Design review of the part built by this model. Coordinates are the model's own, in mm. A direction names the side the tool comes from. Coordinates: 2 decimals unless noted, no trailing zeros. Order: outer loops, then holes, each group sorted by start corner. A loop starts at its lowest first (then second) coordinate and runs counter-clockwise, first axis right, second up. Notation, with made-up numbers: M 53,51 L 107,51 A22 ccw 107,58 Z; hole C 35.5,-28.5 d7. An arc over 180 degrees is marked long. Answer as a JSON object with one key per item and string values.
from build123d import *

# Parameters (mm, degrees)
BOSS_EXTRUDE1_DEPTH     = 150
CUT_EXTRUDE1_DEPTH      = 173.409396496
CUT_EXTRUDE1_DEPTH_BACK = 173.409396496
SKETCH3_OUTSIDE_W       = 197.344
SKETCH3_OUTSIDE_H       = 197.344
BOSS_EXTRUDE2_START     = -80
BOSS_EXTRUDE2_DEPTH     = 80


with BuildPart() as part:
    # Sketch1 → Boss-Extrude1 (new body)
    with BuildSketch(Plane(origin=(0, 0, 0), x_dir=(1, 0, 0), z_dir=(0, 1, 0))):
        with BuildLine():
            Line((-45, -40), (45, -40))
            ThreePointArc((45, -40), (66.213203436, -31.213203436), (75, -10))
            Line((75, -10), (75, 10))
            ThreePointArc((75, 10), (66.213203436, 31.213203436), (45, 40))
            Line((45, 40), (-45, 40))
            ThreePointArc((-45, 40), (-66.213203436, 31.213203436), (-75, 10))
            Line((-75, 10), (-75, -10))
            ThreePointArc((-75, -10), (-66.213203436, -31.213203436), (-45, -40))
        make_face()
    extrude(amount=BOSS_EXTRUDE1_DEPTH)

    # Sketch3 outside → Cut-Extrude1 (cut, two sides: drawn at the far end of the back side and taken through both)
    with BuildSketch(Plane.XY.offset(-CUT_EXTRUDE1_DEPTH_BACK)):
        with Locations((0, 75)):
            Rectangle(SKETCH3_OUTSIDE_W, SKETCH3_OUTSIDE_H)
        with BuildLine():
            Line((-75, 150), (-75, 0))
            Line((-75, 0), (75, 0))
            Line((75, 0), (75, 150))
            ThreePointArc((75, 150), (0, 116.143782777), (-75, 150))
        make_face(mode=Mode.SUBTRACT)
    extrude(amount=CUT_EXTRUDE1_DEPTH + CUT_EXTRUDE1_DEPTH_BACK, mode=Mode.SUBTRACT)

    # Sketch6 → Boss-Extrude2 (add)
    with BuildSketch(Plane.XY.offset(40).offset(BOSS_EXTRUDE2_START)):
        with BuildLine():
            Line((-45, 126.840927279), (-45, 156.143782777))
            ThreePointArc((-45, 156.143782777), (0, 141.143782777), (45, 156.143782777))
            Line((45, 156.143782777), (45, 126.840927279))
            ThreePointArc((45, 126.840927279), (0, 116.143782777), (-45, 126.840927279))
        make_face()
    extrude(amount=BOSS_EXTRUDE2_DEPTH)


solid = part.part
1) Add section D-D (x = -48.5). State the section outline as (y, z) points, and give its area (3 significant figures).
Taken from the geometry:
{"outline": "M 0,-39.8 L 128.69,-39.8 L 128.69,39.8 L 0,39.8 Z", "area": "10,200 mm2"}
2) Mouldability with a two-part tool opening along X and no side actions: class faces 1 (the cylindrical face through (66.445, 73.95, -30.979)), 2 (the flat face through (-45, 141, -1)), 3 (the cylindrical face through (-66.445, 73.95, 30.979)) as released by +X, released by -X, zero draft, split by the parting line, or undercut.
Taken from the geometry:
{"face 1": "released by +X", "face 2": "undercut", "face 3": "released by -X"}
3) Add section C-C (x = -26). State the section outline as (y, z) points.
Taken from the geometry:
{"outline": "M 0,-40 L 145.79,-40 L 145.79,40 L 0,40 Z"}
4) Tool access review of faces 4 (the flat face through (45, 142, -1)), 5 (the flat face through (75, 74, 0)): name each direction out of +Z, -Z, +X, -X, +Y, -Y from which nothing blocks a thin tool from reaching the whole face with its end or side.
Taken from the geometry:
{"face 4": "+Z, -Z, +Y", "face 5": "+Z, -Z, +X, +Y, -Y"}
5) To check wall thickness, follow L1, parallel to X at y = 115.5, z = -10.5; L2, parallel to Z at x = 55.5, y = 79.5; L3, parallel to Y at x = 4, z = 5.5. State the ranges of each line that lie inside material, in increasing order.
Taken from the geometry:
{"L1": "x = -75 to 75", "L2": "z = -38.1 to 38.1", "L3": "y = 0 to 141.25"}
6) Add section A-A (z = -1.5). State the section outline as (x, y) points.
Taken from the geometry:
{"outline": "M -75,0 L 75,0 L 75,150 A100 cw 45,126.84 L 45,156.14 A75 cw -45,156.14 L -45,126.84 A100 cw -75,150 Z"}
7) Insertion check: pin 1 Ø1.5 at (x, z) = (39, 17) entering from +Y; pin 2 Ø10 at (x, z) = (-59, 25.5) entering from +Y; pin 3 Ø6 at (x, z) = (-45, -28) entering from +Y. Each pin has a flat end and moves straight along its axis. Give the tip position at first contact, or say it passes through.
Taken from the geometry:
{"pin 1": "stops at y = 152.54", "pin 2": "stops at y = 139.31", "pin 3": "stops at y = 156.14"}
8) Add section B-B (y = 44). State the section outline as (x, z) points, and give its area (3 significant figures).
Taken from the geometry:
{"outline": "M -75,-10 A30 ccw -45,-40 L 45,-40 A30 ccw 75,-10 L 75,10 A30 ccw 45,40 L -45,40 A30 ccw -75,10 Z", "area": "11,200 mm2"}
